The figure shows three views and two pictorial views of one solid part (mm, origin at its lowest corner). Answer the questions. A direction names the side the tool comes from. Coordinates: 2 decimals unless noted, no trailing zeros. Order: outer loops, then holes, each group sorted by start corner. A loop starts at its lowest first (then second) coordinate and runs counter-clockwise, first axis right, second up. Notation, with made-up numbers: (83.25, 25) -> (131.25, 25) arc R25 cw to (131.25, 62) -> close; hole circle Ø3 at (-11.5, 77.25). An arc over 180 degrees is marked (long way). Return JSON: item names as keys, results as strings.
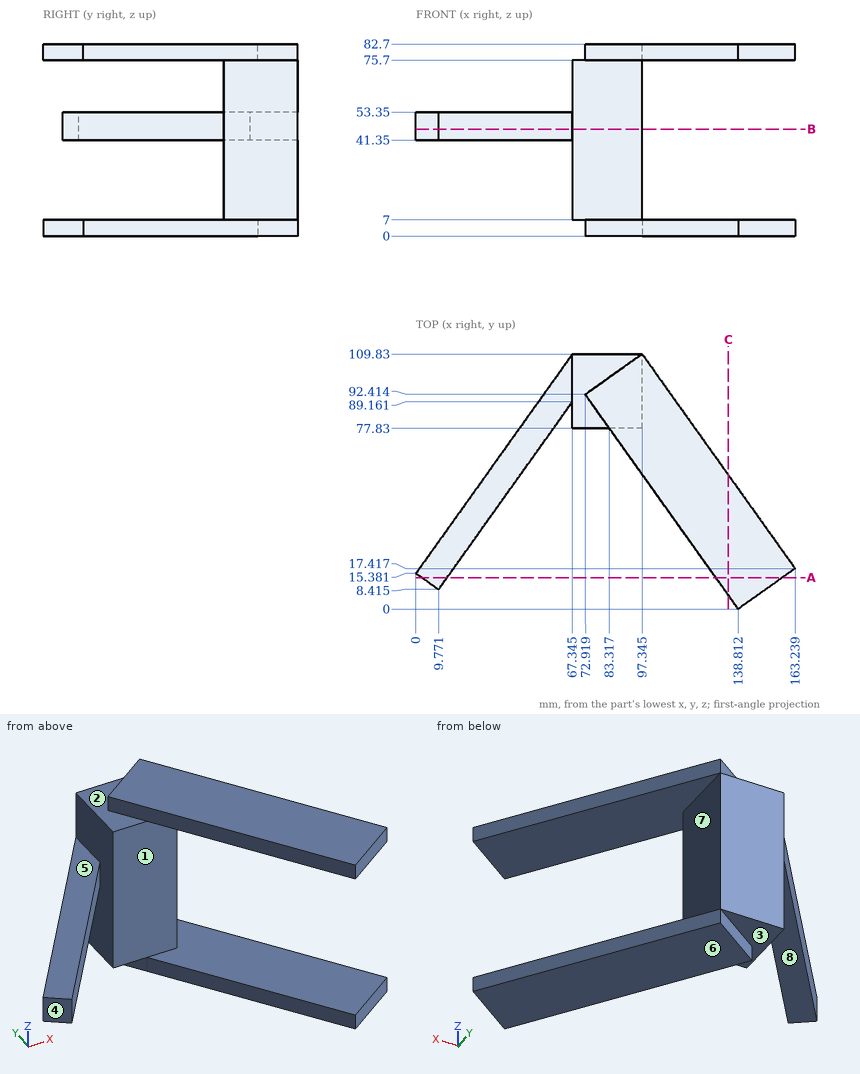
Item 1: Find the intervals of material crossed by probe 1 along Z at (x, y) = (96, 60.5); probe 2 along Z at (x, y) = (37, 61); probe 3 along Y at (x, z) = (72, 62), in increasing order.
Answer list:
{"probe 1": "0 to 7, 75.7 to 82.7", "probe 2": "41.35 to 53.35", "probe 3": "77.83 to 109.83"}
Item 2: Which of the six approach directions +Z, -Z, +X, -X, +Y, -Y give full straight-line access (tool end or side, diameter ignored) to the marked faces 4, 5, 6, 7 and 8?
Answer list:
{"face 4": "+Z, -Z, -X, -Y", "face 5": "+Z, -X, +Y, -Y", "face 6": "-Z, +X, -X, +Y, -Y", "face 7": "+X, +Y, -Y", "face 8": "-Z, -X, +Y, -Y"}
Item 3: The part is cut by section A-A on y = 13.5. Count the separate pieces of the cut face and the enclosed holes in it, plus the area to 3 significant figures.
Answer list:
{"separate pieces": "3", "enclosed holes": "0", "area": "529 mm2"}
Item 4: The part is cut by section B-B on z = 46. Determine the outline of the cut face in (x, y) (1 decimal).
Answer list:
{"outline": "(0, 15.4) -> (9.8, 8.4) -> (67.3, 89.2) -> (67.3, 77.8) -> (97.3, 77.8) -> (97.3, 109.8) -> (67.3, 109.8) -> close"}
Item 5: Determine the mould class of the marked faces 1, 2 and 3 for opening direction Z: pulls with the +Z half, pulls with the -Z half, needs draft (parallel to the pull), parting line crosses it, or undercut.
Answer list:
{"face 1": "undercut", "face 2": "pulls with the +Z half", "face 3": "pulls with the -Z half"}
Item 6: The part is cut by section C-C on x = 134.5. Determine the outline of the cut face in (y, z).
Answer list:
{"outline": "(6.05, 0) -> (57.72, 0) -> (57.72, 7) -> (6.05, 7) -> close; (6.05, 75.7) -> (57.72, 75.7) -> (57.72, 82.7) -> (6.05, 82.7) -> close"}
Item 7: Flat-ended cylindrical pins translate along their axes: pin 1 (6 mm diameter, centred on y = 74, z = 67, fed in from +X); pin 2 (10 mm diameter, centred on y = 36, z = 57.5, fed in from -X) (1 decimal); pin 3 (9.5 mm diameter, centred on y = 93.5, z = 24.5, fed in from -X) (1 decimal); pin 4 (24 mm diameter, centred on x = 82.5, y = 90, fed in from -Z). Find the tip coordinate at first contact, or state that the pin passes through.
Answer list:
{"pin 1": "through", "pin 2": "x = 12.7", "pin 3": "x = 67.3", "pin 4": "z = 0"}
